The figure shows three views and two pictorial views of one solid part (mm, origin at its lowest corner). Answer the questions. Round coordinates to 2 decimals unless told otherwise and drop trailing zeros. Order: outer loops, then holes, each group sorted by start corner. A loop starts at its lowest first (then second) coordinate and runs counter-clockwise, first axis right, second up. Notation, with made-up numbers: (-36, -31.75) -> (2, -31.75) arc R8 ccw to (2, -23.75) -> close; hole circle Ø7 at (-24.75, 60.25). An arc over 180 degrees is marked (long way). Return JSON: item names as keys, results as strings. Group by question number.
(1) The part is cut by section D-D (y = 0.7). Determine the outline of the cut face in (x, z) (1 decimal), plus the area to 3 significant figures.
(2) The part is cut by section B-B (x = 39.5). Determine the outline of the cut face in (y, z).
(3) The part is cut by section C-C (z = 8). Determine the outline of the cut face in (x, y).
(4) This flat-tipped pin is pushed along its axis until it touches: pin 1 (0.9 mm diameter, centred on x = 30.5, y = 2, fed in from +Z) (1 decimal). Where does it stop, or does it pass through?
(5) Consider line 1 (Z direction, x = 31, y = 2.65); line 2 (Z direction, x = 49, y = 0.2) (1 decimal); line 3 (Z direction, x = 56, y = 1.35). Determine where each line is inside the solid, lowest interval first. Write a range as [from, to].
(6) The part is cut by section A-A (x = 19.5). Determine the outline of the cut face in (y, z).
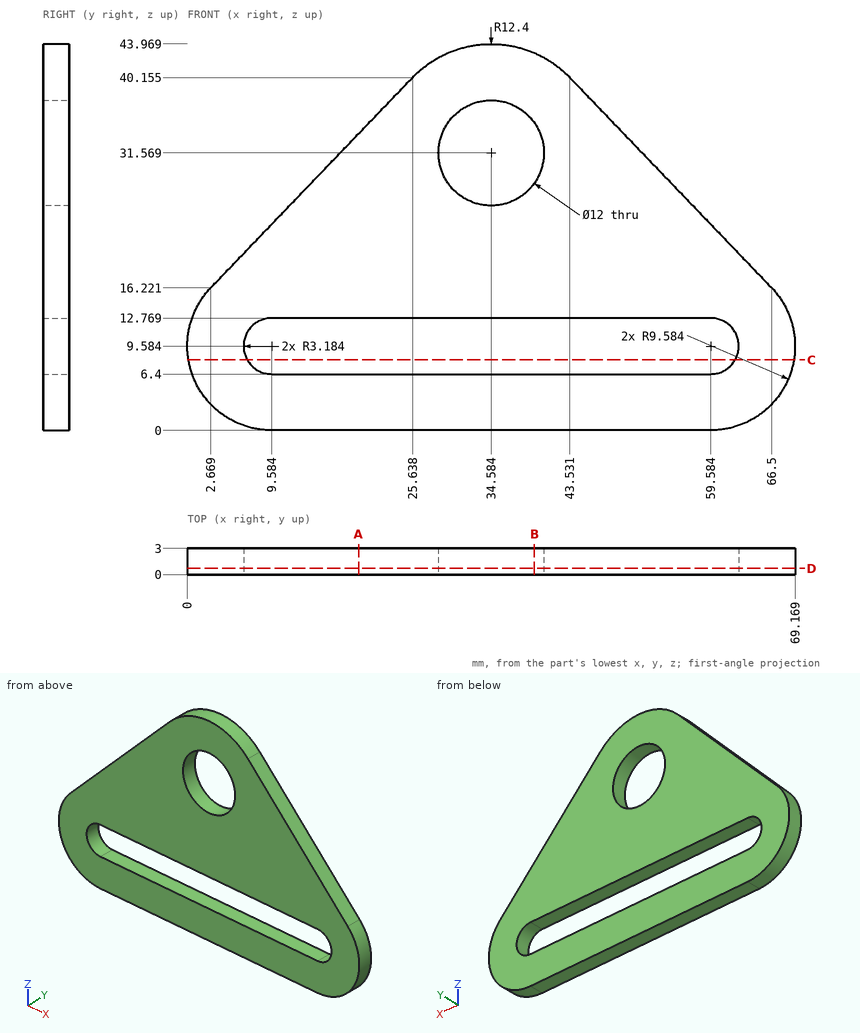
Answer below:
{
 "1": {"outline": "(2.7, 16.2) arc R9.6 ccw to (9.6, 0) -> (59.6, 0) arc R9.6 ccw to (66.5, 16.2) -> (43.5, 40.2) arc R12.4 ccw to (25.6, 40.2) -> close; hole (9.6, 6.4) -> (59.6, 6.4) arc R3.2 ccw to (59.6, 12.8) -> (9.6, 12.8) arc R3.2 ccw to start; hole circle Ø12 at (34.6, 31.6)", "area": "1,630 mm²"},
 "2": {"outline": "(0, 0) -> (3, 0) -> (3, 6.4) -> (0, 6.4) -> close; (0, 12.77) -> (3, 12.77) -> (3, 28.13) -> (0, 28.13) -> close; (0, 35.01) -> (3, 35.01) -> (3, 42.95) -> (0, 42.95) -> close"},
 "3": {"outline": "(0.13, 0) -> (6.82, 0) -> (6.82, 3) -> (0.13, 3) -> close; (62.35, 0) -> (69.04, 0) -> (69.04, 3) -> (62.35, 3) -> close"},
 "4": {"pin 1": "stops at z = 43.4"},
 "5": {"line 1": "z = [0, 6.4], [12.77, 26.76], [36.38, 43.44]", "line 2": "z = [0, 6.4], [12.8, 34.5]", "line 3": "z = [0, 6.4], [12.77, 27.16]"},
 "6": {"outline": "(0, 0) -> (3, 0) -> (3, 6.4) -> (0, 6.4) -> close; (0, 12.77) -> (3, 12.77) -> (3, 33.76) -> (0, 33.76) -> close"}
}
